Autodesk Inventor part; units mm, degrees
ref_plane "YZ Plane" through (0, 0, 0) normal (1, 0, 0) x (0, 1, 0)
ref_plane "XZ Plane" through (0, 0, 0) normal (0, 1, 0) x (-1, 0, 0)
ref_plane "XY Plane" through (0, 0, 0) normal (0, 0, 1) x (1, 0, 0)
sketch "Sketch1" plane through (0, 0, 0) normal (0, 1, 0) x (-1, 0, 0)
  line L0 (29.3688, 15.0812) -> (-29.3688, 15.0812)
  line L1 (-29.3688, 15.0812) -> (-29.3688, -15.0812)
  line L2 (-29.3688, -15.0812) -> (29.3688, -15.0812)
  line L3 (29.3688, -15.0812) -> (29.3688, 15.0812)
  line L4 (41.1163, 0) -> (-41.1162, 0) construction
  line L5 (0, -21.1137) -> (0, 21.1137) construction
  point P0 (0, 0)
  point P1 (0, -15.0812)
  point P2 (29.3688, 0)
  dimension "d0" = 58.7375
  dimension "d1" = 30.1625
extrude "Extrusion1" add sketch "Sketch1" along normal blind 20.6375
sketch "Sketch3" plane through (0, 0, 0) normal (0, 1, 0) x (-1, 0, 0)
  line L0 (-29.3688, 15.0812) -> (-29.3688, -15.0812) construction
  line L1 (41.1163, 0) -> (-41.1163, 0) construction
  line L2 (-29.3688, 9.525) -> (-29.3688, -9.525)
  line L3 (-29.3688, -9.525) -> (-30.9563, -9.525)
  line L4 (-30.9563, -9.525) -> (-35.7126, -6.8071)
  arc A0 (-32.5438, -2.3813) -> (-32.5438, 2.3813) centre (-32.5438, 0) ccw
  line L5 (-32.5438, -2.3813) -> (-36.5125, -2.3813)
  line L6 (-36.5125, -5.4287) -> (-36.5125, -2.3813)
  line L7 (-29.3688, 9.525) -> (-30.9563, 9.525)
  line L8 (-30.9563, 9.525) -> (-35.7126, 6.8071)
  line L9 (-32.5438, 2.3813) -> (-36.5125, 2.3813)
  line L10 (-36.5125, 5.4287) -> (-36.5125, 2.3813)
  arc A1 (-36.5125, -5.4287) -> (-35.7126, -6.8071) centre (-34.925, -5.4287) ccw
  arc A2 (-35.7126, 6.8071) -> (-36.5125, 5.4287) centre (-34.925, 5.4287) ccw
  point P0 (0, 0)
  point P1 (-29.3688, 0)
  point P2 (-36.5125, -6.35)
  point P3 (-30.1625, 0)
  point P4 (-36.5125, 6.35)
  dimension "d4" = 19.05
  dimension "d5" = 1.5875
  dimension "d6" = 7.1437
  dimension "d7" = 6.35
  dimension "d9" = 4.7625
  dimension "d10" = 6.35
  dimension "d11" = 1.5875
  dimension "d12" = 1.5875
extrude "Extrusion2" add sketch "Sketch3" along normal blind 1.5875
mirror "Mirror1" about plane through (0, 0, 0) normal (1, 0, 0) of "Extrusion2"
fillet "Fillet1" radius 1.5875 2 edges at (0, 20.6375, 15.0812) (0, 20.6375, -15.0812)
properties part number "Drok-DC-9v+-to-5v-Converter"
Could you check a few things on this model? Use its own coordinates, in mm. A direction names the side the tool comes from. Give positions to 0.01 mm unless a question says otherwise; leave off trailing zeros. Order: outer loops, then holes, each group sorted by start corner. A loop starts at its lowest first (then second) coordinate and runs counter-clockwise, first axis right, second up. Notation, with made-up numbers: (22, -29) -> (27, -29) arc R28 ccw to (27, 3) -> close; hole circle Ø9 at (-31.5, -13). An arc over 180 degrees is marked (long way). Return JSON: item names as keys, results as strings.
1. Imagine slicing it at B-B on y = 11.75. List the corners of the cut face in (x, z) for me.
Answer list:
{"outline": "(-29.37, -15.08) -> (29.37, -15.08) -> (29.37, 15.08) -> (-29.37, 15.08) -> close"}
2. On a 3-axis mill with a long thin cutter (end or side, diameter ignored), from which of +Z, -Z, +X, -X, +Y, -Y can I reach the whole of each face in a straight line? I mean faces 4 (the flat face through (-31.3, 1.588, 2.3)), 5 (the flat face through (30, 1, 9.525)), 6 (the flat face through (-30, 1, 9.525)), 7 (the flat face through (30, 1.588, 0)). Say none if no direction works.
Answer list:
{"face 4": "+Z, -Z, -X, +Y", "face 5": "+Z, +X, +Y, -Y", "face 6": "+Z, -X, +Y, -Y", "face 7": "+Z, -Z, +X, +Y"}
3. I need wall thicknesses on line 1 (Y direction, x = 29.5, z = 2.5); line 2 (X direction, y = 16.75, z = 5). Which ranges of each line are inside material? Lowest first, please. Write a range as from..to.
Answer list:
{"line 1": "y = 0..1.59", "line 2": "x = -29.37..29.37"}
4. Imagine slicing it at C-C on z = 0. List the corners of the cut face in (x, y) for me.
Answer list:
{"outline": "(-30.16, 0) -> (30.16, 0) -> (30.16, 1.59) -> (29.37, 1.59) -> (29.37, 20.64) -> (-29.37, 20.64) -> (-29.37, 1.59) -> (-30.16, 1.59) -> close"}
5. Thinking about a two-plate mould opening in X: for faces 1 (the flat face through (36.512, 1, -4)), 2 (the cylindrical face through (-0.411, 20.185, -14.604)), 3 (the cylindrical face through (-36.3, 0.78, -6.22)), which applies, pulls with the +X half, pulls with the -X half, needs draft (parallel to the pull), parting line crosses it, or undercut?
Answer list:
{"face 1": "pulls with the +X half", "face 2": "needs draft", "face 3": "pulls with the -X half"}
6. Imagine slicing it at A-A on z = 3.5. List the corners of the cut face in (x, y) for me.
Answer list:
{"outline": "(-36.51, 0) -> (36.51, 0) -> (36.51, 1.59) -> (29.37, 1.59) -> (29.37, 20.64) -> (-29.37, 20.64) -> (-29.37, 1.59) -> (-36.51, 1.59) -> close"}
7. For pin 1 Ø0.5 at (x, y) = (34, 0.5) entering from -Z; pin 2 Ø5.5 at (x, z) = (-34.5, -2.5) entering from +Y; pin 3 Ø0.5 at (x, y) = (34.5, 0.5) entering from +Z; pin 4 Ø2 at (x, z) = (-13, -9) entering from -Y, each with a flat end and sliding along its axis, tell me the tip position at first contact or that it passes through.
Answer list:
{"pin 1": "stops at z = -7.93", "pin 2": "stops at y = 1.59", "pin 3": "stops at z = 7.64", "pin 4": "stops at y = 0"}
